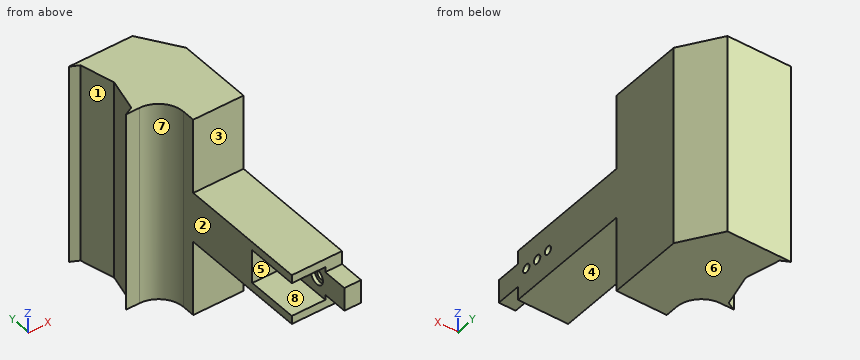
Autodesk Inventor part; units mm, degrees
ref_plane "Work Plane1" through (0, 0, -15) normal (0, 0, 1) x (1, 0, 0)
ref_plane "YZ Plane" through (0, 0, 0) normal (1, 0, 0) x (0, 1, 0)
ref_plane "XZ Plane" through (0, 0, 0) normal (0, 1, 0) x (-1, 0, 0)
sketch "Sketch1" plane through (0, 0, 0) normal (0, 0, 1) x (1, 0, 0)
  line L0 (0, 0) -> (25, 0)
  line L1 (25, 0) -> (25, 40)
  line L2 (25, 40) -> (0, 40)
  line L3 (0, 40) -> (0, 0)
  dimension "d1" = 25
  dimension "d2" = 40
  dimension "d3" = 25
extrude "Extrusion1" add sketch "Sketch1" against normal blind 30
sketch "Sketch2" plane through (25, 0, 0) normal (1, 0, 0) x (0, 0, -1)
  line L0 (0, 0) -> (30, 0)
  circle A0 centre (15, 6.56) radius 2.46
extrude "Extrusion2" cut sketch "Sketch2" against normal blind 30
sketch "Sketch3" plane through (0, 0, 0) normal (-1, 0, 0) x (0, 0, 1)
  line L0 (0, 0) -> (-30, 0)
  line L1 (-25.05, 0) -> (-4.95, 0)
  line L2 (-4.95, 0) -> (-4.95, 33.12)
  line L3 (-4.95, 33.12) -> (-25.05, 33.12)
  line L4 (-25.05, 33.12) -> (-25.05, 0)
  dimension "d11" = 20.1
extrude "Extrusion3" cut sketch "Sketch3" against normal blind 20
sketch "Sketch4" plane through (0, 0, 0) normal (0, -1, 0) x (1, 0, 0)
  line L0 (20, -4.95) -> (20, -25.05)
  line L1 (20, -15) -> (25, -15)
  line L2 (25, 0) -> (25, -30)
  line L3 (20, -8.025) -> (25, -8.025)
  line L4 (25, -8.025) -> (25, -21.975)
  line L5 (25, -21.975) -> (20, -21.975)
  line L6 (20, -21.975) -> (20, -8.025)
  line L7 (20, -8.025) -> (25, -21.975) construction
  line L8 (25, -8.025) -> (20, -21.975) construction
  line L9 (25, -12.54) -> (25, -17.46)
  point P0 (0, 0)
  point P1 (22.5, -15)
  dimension "d14" = 13.95
extrude "Extrusion4" add sketch "Sketch4" along normal blind 15
sketch "Sketch5" plane through (20, 0, 0) normal (-1, 0, 0) x (0, 0, 1)
  circle A0 centre (-15, 6.56) radius 2.46
  circle A1 centre (-15, 6.56) radius 4.7025
  circle A2 centre (-15, 6.56) radius 2.46
  circle A3 centre (-15, 6.56) radius 2.46
  point P0 (0, 0)
  dimension "d17" = 9.405
extrude "Extrusion5" cut sketch "Sketch5" against normal blind 2.1
sketch "Sketch6" plane through (25, 0, 0) normal (1, 0, 0) x (0, 0, -1)
  circle A0 centre (15, 6.56) radius 4.7025
  line L0 (15, 6.56) -> (15, 23.56)
  circle A1 centre (15, 23.56) radius 2.46
  point P0 (0, 0)
  dimension "d20" = 17
  dimension "d21" = 4.92
extrude "Extrusion6" cut sketch "Sketch6" against normal blind 10 contours A1
sketch "Sketch7" plane through (20, 0, 0) normal (-1, 0, 0) x (0, 0, 1)
  circle A0 centre (-15, 23.56) radius 2.46
  circle A1 centre (-15, 23.56) radius 4.7025
  point P0 (0, 0)
  dimension "d24" = 9.405
extrude "Extrusion7" cut sketch "Sketch7" against normal blind 2.1
sketch "Sketch9" plane through (25, 0, 0) normal (1, 0, 0) x (0, 0, -1)
  circle A0 centre (15, 6.56) radius 2.46
  circle A1 centre (15, 6.56) radius 2.46
  circle A2 centre (15, 23.56) radius 2.46
  circle A3 centre (15, 23.56) radius 2.46
  line L0 (30, 40) -> (30, 0)
  line L1 (30, 0) -> (30, 40)
  line L2 (30, 40) -> (0, 40)
  line L3 (0, 40) -> (0, 0)
  line L4 (0, 0) -> (8.025, 0)
  line L5 (21.975, 0) -> (21.975, -15)
  line L6 (21.975, -15) -> (8.025, -15)
  line L7 (8.025, -15) -> (8.025, 0)
  line L8 (0, 0) -> (8.025, 0)
  line L9 (21.975, 0) -> (30, 0)
extrude "Extrusion8" add sketch "Sketch9" along normal blind 5
sketch "Sketch10" plane through (0, 40, 0) normal (0, 1, 0) x (1, 0, 0)
  line L0 (0, 30) -> (30, 30)
  line L1 (30, 0) -> (0, 0)
  line L2 (0, 30) -> (30, 30)
  line L3 (30, 30) -> (30, 0)
  line L4 (30, 0) -> (0, 0)
  line L5 (0, 0) -> (0, 30)
extrude "Extrusion9" add sketch "Sketch10" along normal blind 30
sketch "Sketch12" plane through (30, 0, 0) normal (1, 0, 0) x (0, 0, -1)
  circle A0 centre (15, 6.56) radius 2.46
  line L0 (15, 6.56) -> (15, 15.06)
  circle A1 centre (15, 15.06) radius 2.525
  point P0 (0, 0)
  dimension "d31" = 8.5
  dimension "d33" = 5.05
extrude "Extrusion10" cut sketch "Sketch12" against normal blind 30 contours A1
sketch "Sketch14" plane through (0, 0, 0) normal (0, 0, 1) x (1, 0, 0)
  line L0 (30, 70) -> (0, 70)
  line L1 (0, 70) -> (0, 85)
  line L2 (-15, 100) -> (-23, 100)
  line L3 (30, 0) -> (30, 70)
  line L4 (30, 122.5) -> (30, 70)
  arc A0 (0, 85) -> (-15, 100) centre (-15, 85) ccw
  line L5 (30, 105) -> (30, 100)
  line L6 (-23, 145) -> (15, 145)
  line L7 (-18, 142.5) -> (-23, 145)
  line L8 (-18, 102.5) -> (-23, 100)
  line L9 (-18, 102.5) -> (-13, 122.5)
  line L10 (-13, 122.5) -> (-18, 142.5)
  line L11 (30, 122.5) -> (15, 145)
  point P0 (0, 0)
  point P1 (0, 100)
  dimension "d47" = 30
  dimension "d54" = 15
extrude "Extrusion12" add sketch "Sketch14" against normal blind 30
sketch "Sketch15" plane through (0, 0, -25.05) normal (-1, 0, 0) x (0, 0, 1)
  line L0 (0, 33.12) -> (20.1, 33.12)
  line L1 (20.1, 33.12) -> (20.1, 0)
  line L2 (0, 33.12) -> (20.1, 33.12)
  line L3 (20.1, 33.12) -> (20.1, 31.1)
  line L4 (20.1, 31.1) -> (0, 31.1)
  line L5 (0, 31.1) -> (0, 33.12)
  point P0 (25.05, 0)
  dimension "d57" = 2.02
extrude "Extrusion13" add sketch "Sketch15" against normal blind 20
sketch "Sketch24" plane through (0, 0, 0) normal (0, 0, 1) x (1, 0, 0)
  line L0 (-15, 100) -> (-23, 100)
  line L1 (-15, 100) -> (-23, 100)
  line L2 (-23, 100) -> (-18, 102.5)
  line L3 (-23, 100) -> (-18, 102.5)
  line L4 (-18, 102.5) -> (-13, 122.5)
  line L5 (-18, 102.5) -> (-13, 122.5)
  line L6 (-13, 122.5) -> (-18, 142.5)
  line L7 (-13, 122.5) -> (-18, 142.5)
  line L8 (-18, 142.5) -> (-23, 145)
  line L9 (-18, 142.5) -> (-23, 145)
  line L10 (-23, 145) -> (15, 145)
  line L11 (-23, 145) -> (15, 145)
  line L12 (15, 145) -> (30, 122.5)
  line L13 (15, 145) -> (30, 122.5)
  line L14 (30, 122.5) -> (30, 77.5)
  line L15 (30, 0) -> (30, 122.5)
  line L16 (30, 77.5) -> (0, 77.5)
  line L17 (0, 0) -> (0, 85)
  line L18 (0, 77.5) -> (0, 85)
  arc A0 (0, 85) -> (-15, 100) centre (-15, 85) ccw
  arc A1 (0, 85) -> (-15, 100) centre (-15, 85) ccw
  dimension "d86" = 45
extrude "Extrusion14" add sketch "Sketch24" along normal blind 45
ref_plane "Work Plane1" through (0, 0, -15) normal (0, 0, 1) x (1, 0, 0)
mirror "Mirror1" about plane through (0, 0, -15) normal (0, 0, 1) of "Extrusion14"
properties part number "rec_a_40mm_x_120mm"
The model under review builds one solid part; all positions refer to its coordinate system, in mm. Face numbers are marked on the shaded views. A direction names the side the tool comes from. Round coordinates to 2 decimals unless told otherwise and drop trailing zeros. Order: outer loops, then holes, each group sorted by start corner. A loop starts at its lowest first (then second) coordinate and runs counter-clockwise, first axis right, second up.
(1) Take a section at C-C, the plane z = 11.5. State the section outline as (x, y) points, plus the area to 3 significant figures.
Working result:
outline: (-23, 100) - (-15, 100) arc R15 cw to (0, 85) - (0, 77.5) - (30, 77.5) - (30, 122.5) - (15, 145) - (-23, 145) - (-18, 142.5) - (-13, 122.5) - (-18, 102.5) - close
area: 2,630 mm2
(2) Take a section at B-B, the plane z = -15. Count the separate pieces of the cut face and the enclosed holes in it, plus the area to 3 significant figures.
Working result:
separate pieces: 4
enclosed holes: 0
area: 4,310 mm2
(3) Take a section at D-D, the plane y = 64.5. State the section outline as (x, z) points.
Working result:
outline: (0, -30) - (30, -30) - (30, 0) - (0, 0) - close
(4) Wall thickness on L1, parallel to Y at x = 22, z = -15 (1 decimal); L2, parallel to Z at x = 23, y = 15.06 (3 decimals); L3, parallel to Y at x = 23.75, z = -15 (3 decimals): over which ranges is each line inside the solid? List them lowest first.
Working result:
L1: y = -15 to 1.9, 11.3 to 12.5, 17.6 to 18.9, 28.3 to 134.5
L2: z = -30 to -17.525, -12.475 to 0
L3: y = -15 to 4.1, 9.02 to 12.535, 17.585 to 21.1, 26.02 to 131.875
(5) Take a section at A-A, the plane y = 15.06. State the section outline as (x, z) points (3 decimals).
Working result:
outline: (0, -30) - (30, -30) - (30, -17.525) - (20, -17.525) - (20, -25.05) - (0, -25.05) - close; (0, -4.95) - (20, -4.95) - (20, -12.475) - (30, -12.475) - (30, 0) - (0, 0) - close
(6) Mouldability with a two-part tool opening along Z and no side actions: class the marked faces 6, 7 and 8 as released by +Z, released by -Z, zero draft, split by the parting line, or undercut.
Working result:
face 6: released by -Z
face 7: zero draft
face 8: undercut
(7) For P1, Ø24, axis at x = 8.5, z = 28.5, coming from the -Y side; P2, Ø9, axis at x = -18.5, z = 7, coming from the -Y side; P3, Ø10.5, axis at y = 22, z = -17.5, coming from the -X side, all flat-tipped, find the tip position at first contact; note any pin that passes through.
Working result:
P1: stops at y = 77.5
P2: stops at y = 99.97
P3: stops at x = 20
(8) Tool access review of the marked faces 1, 2, 3, 4 and 5: name each direction out of +Z, -Z, +X, -X, +Y, -Y from which nothing blocks a thin tool from reaching the whole face with its end or side.
Working result:
face 1: +Z, -Z, -X
face 2: +Z, -Z, -X, -Y
face 3: +Z, +X, -X, -Y
face 4: -Z, +X, -X, -Y
face 5: -X, -Y
